Can you work these out from the model? Positions are in its coordinate system, mm. Give positions to 0.01 mm unless a question says otherwise; leave off trailing zeros. Order: outer loops, then holes, each group sorted by start corner. A loop starts at its lowest first (then second) coordinate and runs counter-clockwise, first axis right, second up.
Item 1: If I drill on line 1 along Z through (x, y) = (3.5, 146.08); line 2 along Z through (x, y) = (4.25, 227); line 3 along Y through (x, z) = (2.75, 84), over which ranges is the centre line in solid material (lowest first)?
Item 2: I'm going to push a flat-ended pin straight in: pin 1 Ø2 at (x, z) = (2.5, 56) entering from +Y. Where does the tip first touch, or does it pass through?
Item 3: If we mould it in two halves opening along Z, with no side actions, what happens to faces 1 (the cylindrical face through (3.13, 306.24, -111.42)), 2 (the cylindrical face through (3.13, 233.85, 89.31)), 3 (the flat face through (3.131, 165.996, 46.949))? For each: +Z half, -Z half, draft (parallel to the pull), parting line (faces both ways), or undercut.
Item 4: I want a section at A-A, the plane z = -144.5. Write out the boundary of the cut face in (x, y).
Item 5: I want a section at B-B, the plane x = 2. Count the separate pieces of the cut face and the enclosed holes in it, then the cut area to 3 significant figures.
Autodesk Inventor part; units mm, degrees
ref_plane "YZ Plane" through (0, 0, 0) normal (1, 0, 0) x (0, 1, 0)
ref_plane "XZ Plane" through (0, 0, 0) normal (0, 1, 0) x (-1, 0, 0)
ref_plane "XY Plane" through (0, 0, 0) normal (0, 0, 1) x (1, 0, 0)
sketch "Sketch1" plane through (0, 0, 0) normal (1, 0, 0) x (0, 1, 0)
  line L0 (127, 0) -> (127, -31.75) construction
  line L1 (95.25, -63.5) -> (31.75, -63.5) construction
  line L2 (0, -31.75) -> (0, 0) construction
  arc A0 (95.25, -63.5) -> (127, -31.75) centre (95.25, -31.75) ccw construction
  arc A1 (0, -31.75) -> (31.75, -63.5) centre (31.75, -31.75) ccw construction
  line L3 (0, 0) -> (0, 19.05) construction
  line L4 (0, 19.05) -> (-12.7, 19.05) construction
  line L5 (82.55, 19.05) -> (82.55, 292.1) construction
  circle A2 centre (82.55, 292.1) radius 25.4 construction
  circle A3 centre (82.55, 292.1) radius 31.75 construction
  circle A4 centre (231.775, 292.1) radius 25.4 construction
  circle A5 centre (231.775, 292.1) radius 31.75 construction
  line L6 (-12.7, 19.05) -> (82.55, 19.05) construction
  line L7 (127, 0) -> (0, 0) construction
  line L8 (-12.7, 19.05) -> (-12.7, -285.75) construction
  circle A6 centre (38.1, -172.5837) radius 50.8 construction
  circle A7 centre (104.9083, -202.0677) radius 25.4 construction
  circle A8 centre (104.9083, -202.0677) radius 14.2875
  circle A9 centre (154.8209, -171.8196) radius 25.4 construction
  circle A10 centre (154.8209, -171.8196) radius 14.2875
  circle A11 centre (250.0002, -47.5843) radius 22.225 construction
  circle A12 centre (250.0002, -47.5843) radius 25.4 construction
  circle A13 centre (250.0002, -47.5843) radius 14.2875
  line L9 (82.55, 19.05) -> (127, 19.05) construction
  line L10 (127, 19.05) -> (127, 0) construction
  circle A14 centre (154.8209, -171.8196) radius 22.225 construction
  circle A15 centre (104.9083, -202.0677) radius 22.225 construction
  circle A16 centre (25.4, -99.06) radius 25.4 construction
  circle A17 centre (25.4, -99.06) radius 23.8125 construction
  line L11 (25.4, -73.66) -> (25.4, -63.5) construction
  circle A18 centre (219.8086, -102.3786) radius 25.4 construction
  circle A19 centre (219.8086, -102.3786) radius 22.225 construction
  circle A20 centre (219.8086, -102.3786) radius 14.2875
  line L12 (0, -99.06) -> (-12.7, -99.06) construction
  circle A21 centre (63.172, -79.375) radius 6.477 construction
  circle A22 centre (25.4, -99.06) radius 14.2875
  circle A23 centre (63.172, -79.375) radius 3.2512
  circle A24 centre (95.1707, -129.6948) radius 50.8 construction
  circle A25 centre (147.0613, -96.0158) radius 50.8 construction
  circle A26 centre (105.4747, -117.9903) radius 50.8 construction
  circle A27 centre (166.1747, -221.0415) radius 3.2512
  circle A28 centre (242.3971, 10.8357) radius 14.2875
  circle A29 centre (242.3971, 10.8357) radius 22.225 construction
  line L13 (219.8086, -102.3786) -> (154.8209, -171.8196) construction
  line L14 (154.8209, -171.8196) -> (104.9083, -202.0677) construction
  line L15 (82.55, 19.05) -> (31.75, 19.05) construction
  line L16 (31.75, 19.05) -> (31.75, 292.1) construction
  line L17 (31.75, 292.1) -> (82.55, 292.1) construction
  circle A30 centre (242.3971, 10.8357) radius 7.62 construction
  line L18 (-12.7, -285.75) -> (571.5, -285.75) construction
  line L19 (571.5, -285.75) -> (571.5, 292.1) construction
  line L20 (31.75, 292.1) -> (571.5, 292.1) construction
  line L21 (127, 19.05) -> (571.5, 19.05) construction
  circle A31 centre (230.3321, 82.55) radius 7.62
  circle A32 centre (230.3321, 82.55) radius 23.8125 construction
  circle A33 centre (254.1446, 82.55) radius 2.0828
  circle A34 centre (230.3321, 82.55) radius 27.94 construction
  circle A35 centre (230.3321, 82.55) radius 31.115 construction
  circle A36 centre (242.2384, 103.1722) radius 2.0828
  circle A37 centre (218.4259, 103.1722) radius 2.0828
  circle A38 centre (206.5196, 82.55) radius 2.0828
  circle A39 centre (218.4259, 61.9278) radius 2.0828
  circle A40 centre (242.2384, 61.9278) radius 2.0828
  line L22 (-12.7, -63.5) -> (368.3, -63.5) construction
  circle A41 centre (166.1747, -221.0415) radius 6.4262 construction
  line L23 (368.3, -63.5) -> (368.3, -285.75) construction
  circle A42 centre (63.172, -79.375) radius 6.35 construction
  circle A43 centre (242.3971, 10.8357) radius 25.4 construction
  line L24 (242.3971, 10.8357) -> (250.0002, -47.5843) construction
  line L25 (82.55, 19.05) -> (141.3002, 19.05) construction
  line L26 (141.3002, 19.05) -> (141.3002, 209.55) construction
  line L27 (141.3002, 209.55) -> (82.55, 209.55) construction
  line L28 (82.55, 209.55) -> (82.55, 19.05) construction
  circle A44 centre (133.35, 12.7) radius 6.35 construction
  circle A45 centre (177.4795, -39.017) radius 50.8 construction
  circle A46 centre (177.8, -23.221) radius 50.8 construction
  circle A47 centre (25.4, -99.06) radius 22.225 construction
  line L29 (3.175, -99.06) -> (3.175, -68.2752)
  circle A48 centre (133.35, 12.7) radius 3.2512 construction
  arc A49 (166.1747, -227.4677) -> (170.1786, -226.0679) centre (166.1747, -221.0415) ccw
  arc A50 (3.175, -99.06) -> (20.3984, -120.7149) centre (25.4, -99.06) ccw
  arc A51 (7.9502, -63.5) -> (3.175, -68.2752) centre (7.9502, -68.2752) ccw
  arc A52 (260.5134, 90.1152) -> (205.1617, 100.8419) centre (230.3321, 82.55) ccw
  line L30 (141.3002, 53.086) -> (157.9626, 53.086) construction
  line L31 (157.9626, 53.086) -> (157.9626, 86.106) construction
  line L32 (157.9626, 86.106) -> (141.3002, 86.106) construction
  line L33 (141.3002, 86.106) -> (141.3002, 53.086) construction
  line L34 (232.868, -28.832) -> (267.1324, -66.3365) construction
  circle A53 centre (232.868, -28.832) radius 2.4257
  circle A54 centre (267.1324, -66.3365) radius 2.4257
  line L35 (236.3587, 15.4834) -> (262.5254, -4.6567) construction
  line L36 (236.3587, 15.4834) -> (222.2689, 26.3281) construction
  circle A55 centre (262.5254, -4.6567) radius 2.4257
  circle A56 centre (222.2689, 26.3281) radius 2.4257
  circle A57 centre (262.5254, -4.6567) radius 6.35 construction
  circle A58 centre (222.2689, 26.3281) radius 6.35 construction
  circle A59 centre (232.868, -28.832) radius 6.35 construction
  circle A60 centre (267.1324, -66.3365) radius 6.35 construction
  line L37 (219.8086, -102.3786) -> (237.1646, -83.8332) construction
  line L38 (219.8086, -102.3786) -> (202.4526, -120.9239) construction
  circle A61 centre (237.1646, -83.8332) radius 2.4257
  circle A62 centre (202.4526, -120.9239) radius 2.4257
  circle A63 centre (172.1769, -153.2743) radius 2.4257
  circle A64 centre (133.0985, -184.9838) radius 2.4257
  arc A65 (82.6927, -201.4208) -> (103.7686, -224.2634) centre (104.9083, -202.0677) ccw
  circle A66 centre (9.525, -79.2321) radius 2.4257
  circle A67 centre (9.525, -79.2321) radius 6.35 construction
  arc A68 (82.6927, -201.4208) -> (20.3984, -120.7149) centre (2.2987, -199.0799) ccw
  line L39 (9.525, -79.2321) -> (41.275, -118.8879) construction
  circle A69 centre (41.275, -118.8879) radius 2.4257
  circle A70 centre (41.275, -118.8879) radius 5.6007 construction
  line L40 (7.9502, -63.5) -> (95.25, -63.5)
  arc A71 (95.25, -63.5) -> (127, -31.75) centre (95.25, -31.75) ccw
  line L41 (166.1747, -227.4677) -> (103.7686, -224.2634)
  line L42 (104.9083, -202.0677) -> (83.1859, -215.2319) construction
  line L43 (82.55, 133.35) -> (88.9, 133.35) construction
  line L44 (82.55, 184.15) -> (88.9, 184.15) construction
  line L45 (127, -31.75) -> (127, -8.2637)
  line L46 (127.9123, -5.4564) -> (205.1617, 100.8419)
  arc A72 (127.9123, -5.4564) -> (127, -8.2637) centre (131.7752, -8.2637) ccw
  line L47 (82.55, 44.45) -> (571.5, 44.45) construction
  circle A73 centre (133.0985, -184.9838) radius 6.35 construction
  circle A74 centre (141.7169, -99.98) radius 50.8 construction
  circle A75 centre (277.7476, -102.0288) radius 30 construction
  circle A76 centre (277.7476, -102.0288) radius 25.4 construction
  circle A77 centre (303.1476, -102.0288) radius 2.3876
  circle A78 centre (295.7081, -84.0683) radius 2.3876
  circle A79 centre (277.7476, -76.6288) radius 2.3876 construction
  circle A80 centre (259.7871, -84.0683) radius 2.3876
  circle A81 centre (252.3476, -102.0288) radius 2.3876
  circle A82 centre (259.7871, -119.9893) radius 2.3876
  circle A83 centre (277.7476, -127.4288) radius 2.3876
  circle A84 centre (295.7081, -119.9893) radius 2.3876
  circle A85 centre (277.7476, -102.0288) radius 9.525
  circle A86 centre (219.8086, -102.3786) radius 19.05 construction
  circle A87 centre (227.4601, -139.7023) radius 19.05 construction
  circle A88 centre (227.4601, -139.7023) radius 14.2875
  line L48 (247.7482, -102.2099) -> (245.2082, -102.2252) construction
  line L49 (170.1786, -226.0679) -> (296.4391, -125.4942)
  line L50 (260.5134, 90.1152) -> (306.8474, -94.7347)
  arc A89 (296.4391, -125.4942) -> (306.8474, -94.7347) centre (277.7476, -102.0288) ccw
  circle A90 centre (219.8086, -102.3786) radius 30.48 construction
  circle A91 centre (277.7476, -102.0288) radius 30.48 construction
  circle A92 centre (248.6408, -79.4624) radius 3.81 construction
  line L51 (251.6519, -81.7968) -> (253.6592, -83.3531) construction
  line L52 (245.6582, -81.833) -> (243.6698, -83.4134) construction
  circle A93 centre (248.6408, -79.4624) radius 2.3812
  circle A94 centre (248.9154, -124.945) radius 3.81 construction
  circle A95 centre (248.9154, -124.945) radius 2.3876
  line L53 (251.898, -122.5744) -> (253.8865, -120.9939) construction
  line L54 (245.9043, -122.6105) -> (243.897, -121.0542) construction
  line L55 (248.6408, -75.6524) -> (248.6408, -72.9479) construction
  line L56 (219.8086, -102.3786) -> (219.8086, -88.0911) construction
  circle A96 centre (232.868, -28.832) radius 2.4257
  circle A97 centre (9.525, -79.2321) radius 2.4257
  circle A98 centre (146.08, -220.0775) radius 2.4257
  circle A99 centre (253.6387, -151.4689) radius 2.4257
  circle A100 centre (209.9304, -186.285) radius 2.4257
  circle A101 centre (281.6771, -62.9926) radius 2.4257
  line L57 (123.7263, -57.0623) -> (232.868, -28.832) construction
  line L58 (232.868, -28.832) -> (281.6771, -62.9926) construction
  line L59 (281.6771, -62.9926) -> (253.6387, -151.4689) construction
  line L60 (253.6387, -151.4689) -> (209.9304, -186.285) construction
  line L61 (209.9304, -186.285) -> (146.08, -220.0775) construction
  line L62 (146.08, -220.0775) -> (9.525, -79.2321) construction
  line L63 (123.7263, -57.0623) -> (9.525, -79.2321) construction
  circle A102 centre (146.08, -220.0775) radius 6.35 construction
  circle A103 centre (123.7263, -57.0623) radius 2.4257
  line L64 (277.7476, -102.0288) -> (219.8086, -102.3786) construction
  line L65 (250.0002, -47.5843) -> (219.8086, -102.3786) construction
  point P0 (-12.7, -172.5837)
  point P1 (180.2209, -171.8196)
  point P2 (104.775, 19.05)
  point P3 (172.6009, -221.0415)
  point P4 (127, -63.5)
  point P5 (3.175, -63.5)
  point P6 (104.9083, -227.4677)
  point P7 (95.25, -63.5)
  point P8 (127, -6.7118)
  point P9 (222.7121, 82.55)
  point P10 (220.1721, 10.8357)
  point P11 (25.4, -99.06)
  dimension "d58" = 101.6
  dimension "d267" = 15.24
  dimension "d283" = 15.24
  dimension "d284" = 47.625
  dimension "d523" = 50.8
  dimension "d2" = 31.75
  dimension "d3" = 19.05
  dimension "d4" = 12.7
  dimension "d7" = 273.05
  dimension "d8" = 50.8
  dimension "d9" = 6.35
  dimension "d10" = 50.8
  dimension "d11" = 6.35
  dimension "d12" = 149.225
  dimension "d14" = 127
  dimension "d16" = 304.8
  dimension "d175" = 31.75
  dimension "d180" = 50.8
  dimension "d181" = 1.5875
  dimension "d187" = 31.75
  dimension "d189" = 12.7
  dimension "d191" = 12.954
  dimension "d192" = 28.575
  dimension "d201" = 6.5024
  dimension "d207" = 101.6
  dimension "d208" = 101.6
  dimension "d210" = 130.175
  dimension "d214" = 15.875
  dimension "d218" = 6.5024
  dimension "d220" = 143.1895
  dimension "d236" = 50.8
  dimension "d237" = 44.45
  dimension "d271" = 584.2
  dimension "d285" = 4.1656
  dimension "d290" = 55.88
  dimension "d292" = 3.175
  dimension "d321" = 360
  dimension "d323" = 381
  dimension "d328" = 3.175
  dimension "d336" = 12.7
  dimension "d375" = 10.16
  dimension "d388" = 50.8
  dimension "d389" = 3.175
  dimension "d395" = 44.45
  dimension "d399" = 58.7502
  dimension "d400" = 190.5
  dimension "d404" = 12.7
  dimension "d405" = 101.6
  dimension "d406" = 101.6
  dimension "d409" = 3.175
  dimension "d410" = 6.5024
  dimension "d411" = 4.7752
  dimension "d427" = 16.6624
  dimension "d428" = 33.02
  dimension "d429" = 34.036
  dimension "d433" = 4.8514
  dimension "d434" = 4.8514
  dimension "d435" = 4.8514
  dimension "d436" = 4.8514
  dimension "d441" = 45
  dimension "d443" = 4.8514
  dimension "d444" = 4.8514
  dimension "d445" = 4.8514
  dimension "d446" = 4.8514
  dimension "d453" = 4.8514
  dimension "d459" = 4.8514
  dimension "d460" = 3.175
  dimension "d470" = 273.05
  dimension "d471" = 62.5615
extrude "Extrusion14" add sketch "Sketch1" along normal blind 6.35 contours L29 A51 L40 A71 L45 A72 L46 A52 L50 A89 L49 A49 L41 A65 A68 A50 | A77 | A81 | A83 | A93 | A95 | A98 | A99 | A100 | A101 | A103
extrude "Extrusion15" cut sketch "Sketch1" along normal blind 6.35 contours A77 | A81 | A83
extrude "Extrusion16" cut sketch "Sketch1" along normal blind 6.35 contours A93 | A95
extrude "Extrusion17" cut sketch "Sketch1" along normal blind 25.4 contours A98 | A99 | A100 | A101 | A103
properties part number "Intake Roller Plate" material "Aluminum 6061"
Results list:
1. line 1: z = -226.44 to -222.5, -217.65 to -183.12, -160.52 to 19.54
1. line 2: z = -180.81 to -153.98, -125.42 to -114.72, -90.03 to 75.7, 89.4 to 113.49
1. line 3: y = 192.92 to 205.02, 208.01 to 222.85, 237.81 to 252.65, 255.64 to 262.05
2. pin 1: stops at y = 269.32
3. face 1: parting line
3. face 2: undercut
3. face 3: +Z half
4. outline: (0, 61.37) - (6.35, 61.37) - (6.35, 214) - (0, 214) - close; (0, 240.92) - (6.35, 240.92) - (6.35, 272.58) - (0, 272.58) - close
5. separate pieces: 1
5. enclosed holes: 41
5. area: 50,200 mm2
